from build123d import *

# Parameters (mm, degrees)
F0_W     = 30
F0_H     = 60
F0_R     = 1
F0_R_2   = 6.25
F1_DEPTH = 1.5
F2_W     = 30
F2_H     = 1.5
F3_DEPTH = 10
F4_R     = 1
F5_DEPTH = 60.001
F6_W     = 57
F6_H     = 1.5
F7_DEPTH = 4


with BuildPart() as f1:
    # F0 (on Top) → F1 (new body)
    with BuildSketch(Plane.XY):
        with Locations((0, 10)):
            Rectangle(F0_W, F0_H)
        with Locations((-10.5, -11)):
            Circle(F0_R, mode=Mode.SUBTRACT)
        with Locations((10.5, -11)):
            Circle(F0_R, mode=Mode.SUBTRACT)
        with Locations((-10.5, 10)):
            Circle(F0_R, mode=Mode.SUBTRACT)
        with Locations((-10.5, 31)):
            Circle(F0_R, mode=Mode.SUBTRACT)
        with Locations((0, 10)):
            Circle(F0_R_2, mode=Mode.SUBTRACT)
        with Locations((10.5, 10)):
            Circle(F0_R, mode=Mode.SUBTRACT)
        with Locations((10.5, 31)):
            Circle(F0_R, mode=Mode.SUBTRACT)
    extrude(amount=F1_DEPTH)

    # F2 (on face) → F3 (join)
    with BuildSketch(Plane.XY.offset(1.5)):
        with Locations((0, 39.25)):
            Rectangle(F2_W, F2_H)
        with Locations((0, -19.25)):
            Rectangle(F2_W, F2_H)
    extrude(amount=F3_DEPTH)

    # F4 (on face) → F5 (cut, through all)
    with BuildSketch(Plane(origin=(0, 40, 0), x_dir=(-1, 0, 0), z_dir=(0, 1, 0))):
        with Locations((-10, 7.5)):
            Circle(F4_R)
        with Locations((10, 7.5)):
            Circle(F4_R)
    extrude(amount=-F5_DEPTH, mode=Mode.SUBTRACT)

    # F6 (on face) → F7 (join)
    with BuildSketch(Plane.YZ.offset(15)):
        with Locations((10, 0.75)):
            Rectangle(F6_W, F6_H)
    extrude(amount=F7_DEPTH)


solid = f1.part
Geometry check sheet. Reference: the model listing, model coordinates, mm. A direction names the side the tool comes from. Round coordinates to 2 decimals unless told otherwise and drop trailing zeros. Loops run counter-clockwise (first coordinate to the right, second up) from the corner with the lowest first, then second, coordinate; pieces in that order, holes last. Notation, with made-up numbers: (46, -17) - (73, -17) arc R33 ccw to (73, 19) - close; hole circle Ø9 at (26.5, 59.25). An arc over 180 degrees is marked (long way). Answer as CSV lines item,"result".
(1) Cross-section at D-D, the plane y = 31. Enter the section's corners in (x, z).
Output values:
outline,"(-15, 0) - (-11.5, 0) - (-11.5, 1.5) - (-15, 1.5) - close; (-9.5, 0) - (9.5, 0) - (9.5, 1.5) - (-9.5, 1.5) - close; (11.5, 0) - (19, 0) - (19, 1.5) - (11.5, 1.5) - close"
(2) Depth check by flat-ended pin: pin 1 Ø1.8 at (x, y) = (-10.5, 31) entering from +Z; pin 2 Ø10 at (x, y) = (12, -8.5) entering from +Z; pin 3 Ø0.8 at (x, z) = (17, 1) entering from -Y. Enter the tip coordinate at first touch or a pass-through.
Output values:
pin 1,"passes through"
pin 2,"stops at z = 1.5"
pin 3,"stops at y = -18.5"
(3) Cross-section at C-C, the plane x = 0. Enter the section's corners in (y, z), and give its area (3 significant figures).
Output values:
outline,"(-20, 0) - (3.75, 0) - (3.75, 1.5) - (-18.5, 1.5) - (-18.5, 11.5) - (-20, 11.5) - close; (16.25, 0) - (40, 0) - (40, 11.5) - (38.5, 11.5) - (38.5, 1.5) - (16.25, 1.5) - close"
area,"101 mm²"
(4) Release check for a two-part mould opening along X. For faces 1 (the face through (17, 38.5, 1)), 2 (the face through (-9.87, 39.26, 8.49)), 3 (the face through (-15, 10, 1)) record: released by +X, released by -X, zero draft, split by the parting line, or undercut.
Output values:
face 1,"zero draft"
face 2,"undercut"
face 3,"released by -X"
(5) Cross-section at A-A, the plane y = 10. Enter the section's corners in (x, z), and give its area (4 significant figures).
Output values:
outline,"(-15, 0) - (-11.5, 0) - (-11.5, 1.5) - (-15, 1.5) - close; (-9.5, 0) - (-6.25, 0) - (-6.25, 1.5) - (-9.5, 1.5) - close; (6.25, 0) - (9.5, 0) - (9.5, 1.5) - (6.25, 1.5) - close; (11.5, 0) - (19, 0) - (19, 1.5) - (11.5, 1.5) - close"
area,"26.25 mm²"
(6) Set-up check for faces 4 (the face through (2, 3, 1.5)), 5 (the face through (0, -19, 11.5)): record each of +Z, -Z, +X, -X, +Y, -Y from which the full face is reachable in a straight line by a thin tool's end or side.
Output values:
face 4,"+Z, +X, -X"
face 5,"+Z, +X, -X, +Y, -Y"
(7) Material ranges on line 1 along Y through (x, z) = (1, 2.75); line 2 along Y through (x, z) = (-10.5, 0.5); line 3 along Y through (x, z) = (0, 0.6), recorded low to high.
Output values:
line 1,"y = -20 to -18.5, 38.5 to 40"
line 2,"y = -20 to -12, -10 to 9, 11 to 30, 32 to 40"
line 3,"y = -20 to 3.75, 16.25 to 40"
(8) Cross-section at B-B, the plane z = 3. Enter the section's corners in (x, y), and give its area (3 significant figures).
Output values:
outline,"(-15, -20) - (15, -20) - (15, -18.5) - (-15, -18.5) - close; (-15, 38.5) - (15, 38.5) - (15, 40) - (-15, 40) - close"
area,"90.0 mm²"
